from build123d import *
from build123d.topology import SkipClean

# Parameters (mm, degrees)
SKETCH_3_R                 = 4.85
CUT_EXTRUDE_496_DEPTH      = 38.7
CUT_EXTRUDE_713_DEPTH      = 70.85
PATTERN_CIRCULAR_762_COUNT = 5
SKETCH_5_R                 = 7.5
SKETCH_5_R_2               = 4.85
EXTRUDE_884_DEPTH          = 5
CUT_EXTRUDE_START          = -0.1
CUT_EXTRUDE_1190_DEPTH     = 0.1
FILLET_2_R                 = 2
SKETCH_7_R                 = 1.75
CUT_EXTRUDE_1_DEPTH        = 4


with BuildPart() as part:
    # Эскиз2 → Revolve 372 (revolve)
    with BuildSketch(Plane.XY, mode=Mode.PRIVATE) as revolve_372_sk:
        with BuildLine():
            Line((0, 0), (-48, 0))
            Line((-48, 0), (-48, -50))
            Line((-48, -50), (-46, -50))
            Line((-46, -50), (-46, -5.5))
            ThreePointArc((-46, -5.5), (-45.121320344, -3.378679656), (-43, -2.5))
            Line((-43, -2.5), (0, -2.5))
            Line((0, -2.5), (0, 0))
        make_face()
    revolve(revolve_372_sk.sketch.rotate(Axis((0, 0, 0), (0, 1, 0)), 270), axis=Axis((0, 0, 0), (0, 1, 0)))

    # Эскиз3 → Cut-Extrude 496 (cut)
    with BuildSketch(Plane(origin=(0, 0, 0), x_dir=(1, 0, 0), z_dir=(0, 1, 0))):
        with Locations(Location((0, -10, 0), (0, 0, 270))):
            Circle(SKETCH_3_R)
    extrude(amount=-CUT_EXTRUDE_496_DEPTH, mode=Mode.SUBTRACT)

    # Эскиз4 → Cut-Extrude 713 (cut, symmetric)
    with BuildSketch(Plane.XY):
        Polygon((-6, -7), (6, -7), (0, -37), align=None)
    cut_extrude_713 = extrude(amount=CUT_EXTRUDE_713_DEPTH, both=True, mode=Mode.SUBTRACT)

    # Pattern Circular 762: Cut-Extrude 713 ×5 about axis
    pattern_circular_762_axis = Axis((0, 0, 0), (0, 1, 0))
    for i in range(1, PATTERN_CIRCULAR_762_COUNT):
        add(cut_extrude_713.rotate(pattern_circular_762_axis, i * 360 / PATTERN_CIRCULAR_762_COUNT), mode=Mode.SUBTRACT)

    # Эскиз5 → Extrude 884 (add)
    with BuildSketch(Plane.XZ.offset(2.5)):
        with Locations(Location((0, 10, 0), (0, 0, 90))):
            Circle(SKETCH_5_R)
        with Locations(Location((0, 10, 0), (0, 0, 90))):
            Circle(SKETCH_5_R_2, mode=Mode.SUBTRACT)
    extrude(amount=EXTRUDE_884_DEPTH)

    # Эскиз6 → Cut-Extrude 1190 (cut)
    with SkipClean():  # the faces are left unmerged after this step: merging them gives an invalid solid
        with BuildSketch(Plane.XZ.offset(2.5).offset(CUT_EXTRUDE_START)):
            with BuildLine():
                Line((-0.25, 2.504167825), (-0.25, -34.997321394))
                Line((-0.25, -34.997321394), (0.25, -34.997321394))
                Line((0.25, -34.997321394), (0.25, 2.504167825))
                ThreePointArc((0.25, 2.504167825), (0, 2.5), (-0.25, 2.504167825))
            make_face()
        extrude(amount=CUT_EXTRUDE_1190_DEPTH, mode=Mode.SUBTRACT)

    # Скругление2
    fillet_2_edges = [part.edges().sort_by_distance(p)[0] for p in [
        (0, -7.5, 2.5),
    ]]
    fillet(fillet_2_edges, radius=FILLET_2_R)

    # Эскиз7 → Вырез-Вытянуть1 (cut, symmetric)
    with SkipClean():  # the faces are left unmerged after this step: merging them gives an invalid solid
        with BuildSketch(Plane(origin=(0, 0, 0), x_dir=(1, 0, 0), z_dir=(0, 1, 0))):
            with Locations(Location((44, 0, 0), (0, 0, 234.209624239))):
                Circle(SKETCH_7_R)
            with Locations(Location((-44, 0, 0), (0, 0, 305.790375763))):
                Circle(SKETCH_7_R)
        extrude(amount=CUT_EXTRUDE_1_DEPTH, both=True, mode=Mode.SUBTRACT)


solid = part.part
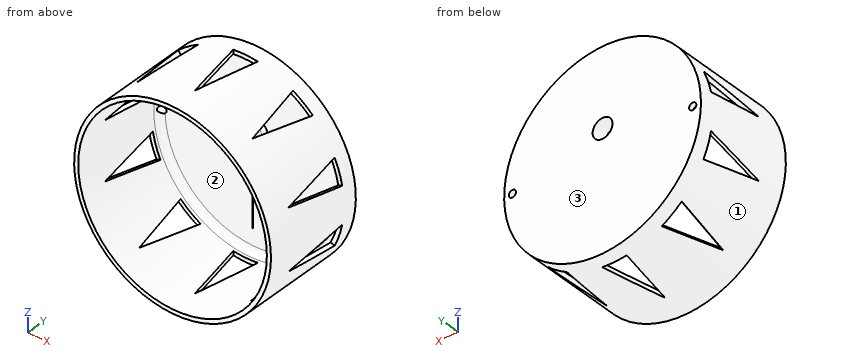
Model file for the job. Use its own axes, mm. Face numbers are marked on the shaded views. Give positions to 0.01 mm unless a question says otherwise; leave off trailing zeros. Use one line per item in the form item = value.
(1) Drill centre lines: L1, parallel to X at y = -1.65, z = 0; L2, parallel to X at y = -23.5, z = 0; L3, parallel to X at y = -2.95, z = 0. Where is each one in solid material? Low to high.
Determined:
L1 = -48 to -45.75, -42.25 to 42.25, 45.75 to 48
L2 = -48 to -46, 46 to 48
L3 = -48 to -45.75, 45.75 to 48
(2) Cut at A-A (x = -30). Count the separate pieces of the cut face and the enclosed holes in it, then the cut area to 3 significant figures.
Determined:
separate_pieces = 3
enclosed_holes = 0
area = 362 mm^2
(3) Drop flat-ended pins along their axis: P1, Ø2, axis at x = 9.5, y = -18.5, coming from the +Z side; P2, Ø3, axis at x = 44, z = -13, coming from the -Y side; P3, Ø4, axis at x = 16, z = 13.5, coming from the -Y side; P4, Ø1.5, axis at x = -34.5, y = -30, coming from the +Z side. Give the stop position or say it passes through.
Determined:
P1 = 47.24
P2 = -50
P3 = -2.5
P4 = 34.13
(4) Pull direction Z, two halves, no side cores. Call the marked faces 1, 2 and 3: pulls with the +Z half, pulls with the -Z half, needs draft (parallel to the pull), parting line crosses it, or undercut.
Determined:
face_1 = parting line crosses it
face_2 = undercut
face_3 = needs draft
